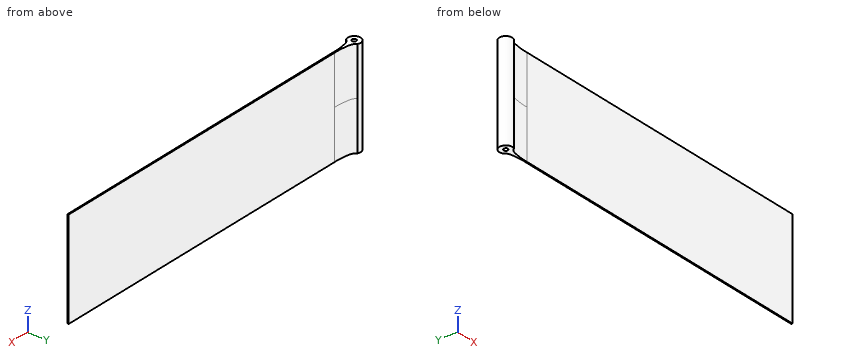
from build123d import *

# Parameters (mm, degrees)
ESQUISSE2_R             = 0.5
BOSS_EXTRU_1_DEPTH      = 11.4
BOSS_EXTRU_1_DEPTH_BACK = 11.4


with BuildPart() as part:
    # Esquisse2 → Boss.-Extru.1 (new body, two sides)
    with BuildSketch(Plane.XY) as boss_extru_1_sk:
        with BuildLine():
            Line((5.791060422, 0.142064292), (80.791060422, 0.133235508))
            ThreePointArc((80.791060422, 0.133235508), (80.791208073, 0), (80.791060422, -0.133235508))
            Line((80.791060422, -0.133235508), (5.791060422, -0.142064292))
            add(Edge.make_bspline(
                [(0.650938463, -1.351398948), (1.114517622, -0.510365175), (3.069897688, -0.268204079), (5.029284194, -0.087299538), (5.791060422, -0.142064292)],
                knots=[0, 0, 0, 0, 0.614720571, 1, 1, 1, 1], degree=3))
            ThreePointArc((0.650938463, -1.351398948), (-1.5, 0), (0.650938463, 1.351398948))
            add(Edge.make_bspline(
                [(0.650938463, 1.351398948), (1.114517622, 0.510365175), (3.069897688, 0.268204079), (5.029284194, 0.087299538), (5.791060422, 0.142064292)],
                knots=[0, 0, 0, 0, 0.614720571, 1, 1, 1, 1], degree=3))
        make_face()
        Circle(ESQUISSE2_R, mode=Mode.SUBTRACT)
    extrude(amount=BOSS_EXTRU_1_DEPTH)
    extrude(boss_extru_1_sk.sketch, amount=-BOSS_EXTRU_1_DEPTH_BACK)


solid = part.part
Source: CAD feature listing. Evaluate the final solid. Frame: model axes, mm. Give positions to 0.01 mm unless a question says otherwise; leave off trailing zeros. Write each loop counter-clockwise with the first axis right and the second up, starting at its lowest first coordinate (ties: lowest second). Pieces come first, ordered by that corner, then holes. Notation, with made-up numbers: M 52,8.25 L 80,8.25 A27 ccw 80,33.25 Z; hole C -1.75,-8.75 d2. An arc over 180 degrees is marked long. Return JSON: item names as keys, results as strings. Group by question number.
1) Cut plane B-B, the plane x = 55.5. Output: boundary loops of the cut face in (y, z), then the cut area to 3 significant figures.
2) Cut plane A-A, the plane x = 71. Output: boundary loops of the cut face in (y, z).
3) First-contact query: pin 1 Ø1 at (x, z) = (30, 4.5) entering from +Y; pin 2 Ø12 at (x, z) = (14.5, 6) entering from -Y. Flat tips, straight axial feed; report the tip coordinate or a pass-through.
4) Ray query, L1, parallel to Y at x = 0, z = 5; L2, parallel to Y at x = 10, z = 1; L3, parallel to X at y = -0.65, z = -6.75. Return the intervals inside material, ascending.
Data:
{
 "1": {"outline": "M -0.14,-11.4 L 0.14,-11.4 L 0.14,11.4 L -0.14,11.4 Z", "area": "6.21 mm²"},
 "2": {"outline": "M -0.13,-11.4 L 0.13,-11.4 L 0.13,11.4 L -0.13,11.4 Z"},
 "3": {"pin 1": "stops at y = 0.14", "pin 2": "stops at y = -0.14"},
 "4": {"L1": "y = -1.5 to -0.5, 0.5 to 1.5", "L2": "y = -0.14 to 0.14", "L3": "x = -1.35 to 1.47"}
}
